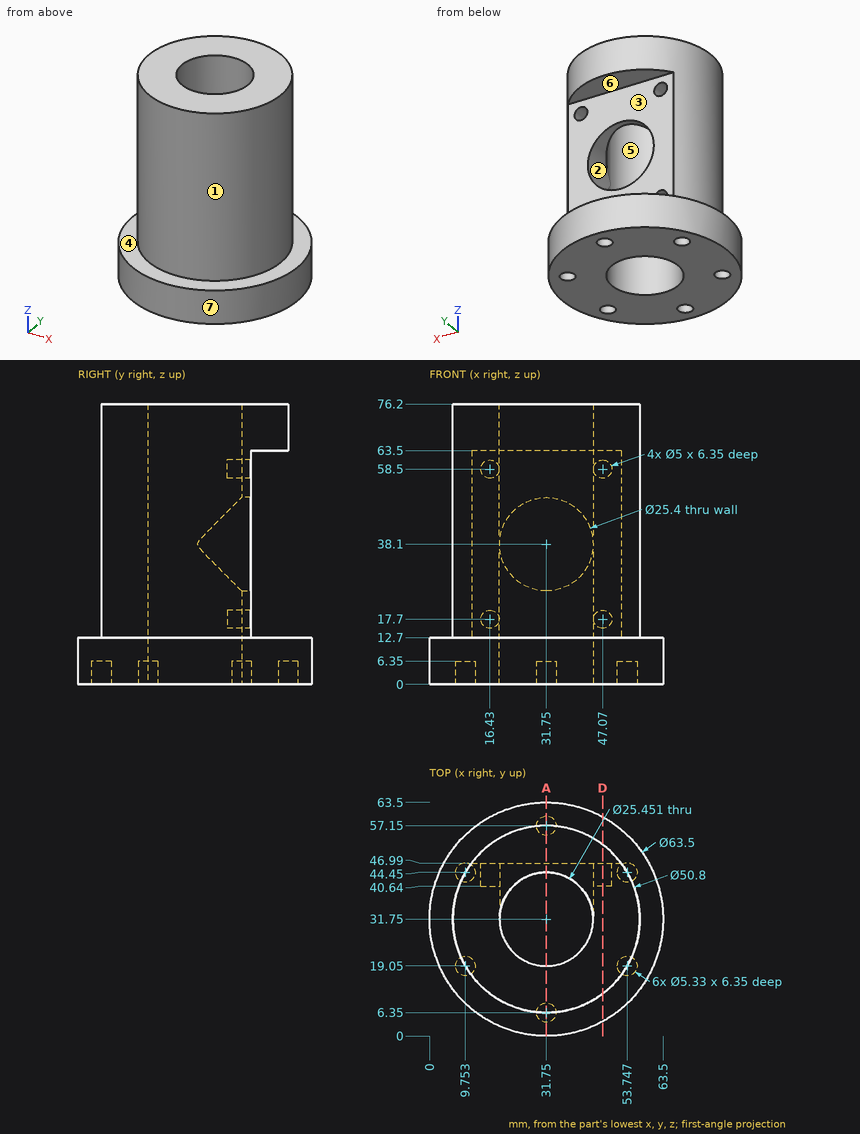
Geometry check sheet. Reference: drawing and pictorial views, mm from the part's lowest x, y, z. A direction names the side the tool comes from. Round coordinates to 2 decimals unless told otherwise and drop trailing zeros. Loops run counter-clockwise (first coordinate to the right, second up) from the corner with the lowest first, then second, coordinate; pieces in that order, holes last. Notation, with made-up numbers: (64, 55) - (106, 55) arc R31 cw to (106, 83) - close; hole circle Ø5 at (52, 1.25). An arc over 180 degrees is marked (long way). Use a Markdown table: item, result. Add a question column.
1. Thickness scan on probe 1 along Z at (x, y) = (31, 47.5); probe 2 along Z at (x, y) = (47, 42); probe 3 along X at (y, z) = (45.75, 58.5). Record the ranges inside material, lowest first. Write a range as [from, to].
2. Gauge pin test, flat ends, axial feed: pin 1 (5.5 mm diameter, centred on x = 46, z = 58.5, fed in from +Y); pin 2 (6 mm diameter, centred on x = 24.5, z = 29.5, fed in from -Y); pin 3 (6 mm diameter, centred on y = 37, z = 9.5, fed in from -X). Record the tip position at first contact, or that the pin passes through.
3. Section check A-A, the plane x = 31.75. Give the number of separate pieces and of enclosed holes in the cut face, plus the area to 3 significant figures.
4. Access from +Z, -Z, +X, -X, +Y, -Y to the whole of each face (thin tool, end or side, straight path). Record for the marked faces 1, 2, 3 and 4.
5. Section check D-D, the plane x = 47.07. Record the boundary of the cut face in (y, z), plus the area to 3 significant figures.
6. Release check for a two-part mould opening along X. For the marked faces 5, 6 and 7 record: released by +X, released by -X, zero draft, split by the parting line, or undercut.
Checks:
| question | item | result |
|---|---|---|
| 1 | probe 1 | z = [0, 12.7], [63.5, 76.2] |
| 1 | probe 2 | z = [0, 15.2], [20.2, 56], [61, 76.2] |
| 1 | probe 3 | x = [10.56, 13.93], [18.93, 44.57], [49.57, 52.94] |
| 2 | pin 1 | stops at y = 46.99 |
| 2 | pin 2 | stops at y = 6.71 |
| 2 | pin 3 | stops at x = 0.08 |
| 3 | separate pieces | 3 |
| 3 | enclosed holes | 0 |
| 3 | area | 1,450 mm^2 |
| 4 | face 1 | +Z |
| 4 | face 2 | +Y |
| 4 | face 3 | +X, -X, +Y |
| 4 | face 4 | none |
| 5 | outline | (3.94, 0) - (59.56, 0) - (59.56, 12.7) - (46.99, 12.7) - (46.99, 15.2) - (40.64, 15.2) - (40.64, 20.2) - (46.99, 20.2) - (46.99, 56) - (40.64, 56) - (40.64, 61) - (46.99, 61) - (46.99, 63.5) - (52.01, 63.5) - (52.01, 76.2) - (11.49, 76.2) - (11.49, 12.7) - (3.94, 12.7) - close |
| 5 | area | 2,960 mm^2 |
| 6 | face 5 | undercut |
| 6 | face 6 | zero draft |
| 6 | face 7 | split by the parting line |
